The model under review builds one solid part; all positions refer to its coordinate system, in mm. A direction names the side the tool comes from. Give positions to 0.01 mm unless a question says otherwise; leave off trailing zeros. Order: outer loops, then holes, each group sorted by start corner. A loop starts at its lowest first (then second) coordinate and runs counter-clockwise, first axis right, second up. Notation, with made-up numbers: (-32.75, 12.5) - (23.25, 12.5) arc R18 cw to (23.25, 32.5) - close; hole circle Ø4 at (-8.5, 79.5). An arc over 180 degrees is marked (long way). Use CSV: the item, a comma, the result in double quotes.
```python
from build123d import *

# Parameters (mm, degrees)
F0_W     = 12.446
F0_H     = 6.096
F1_DEPTH = 5.715
F2_W     = 12.446
F2_H     = 8.509
F3_DEPTH = 10.414
F4_R     = 0.762
F7_D     = 7.874
F7_DEPTH = 6.605


with BuildPart() as f1:
    # F0 (on Top) → F1 (new body)
    with BuildSketch(Plane.XY):
        Rectangle(F0_W, F0_H)
    extrude(amount=F1_DEPTH)

    # F2 (on Top) → F3 (join)
    with BuildSketch(Plane.XY):
        Rectangle(F2_W, F2_H)
    extrude(amount=-F3_DEPTH)

    # F4
    f4_edges = [f1.edges().sort_by_distance(p)[0] for p in [
        (6.223, 0, 5.715),
        (0, 3.048, 5.715),
        (-6.223, 0, 5.715),
        (0, -3.048, 5.715),
    ]]
    fillet(f4_edges, radius=F4_R)

    # F7 (through all, one way)
    with BuildSketch(Plane.XY.offset(-3.81)):
        with Locations((0, 0)):
            Circle(F7_D / 2)
    extrude(amount=-F7_DEPTH, mode=Mode.SUBTRACT)


solid = f1.part
```
Item 1: Tool access review of faces 5 (the face through (0, -4, 0)), 6 (the face through (0, 4, 0)), 7 (the face through (0, 4.254, -5)): name each direction out of +Z, -Z, +X, -X, +Y, -Y from which nothing blocks a thin tool from reaching the whole face with its end or side.
Results list:
face 5,"+Z, +X, -X, -Y"
face 6,"+Z, +X, -X, +Y"
face 7,"+Z, -Z, +X, -X, +Y"
Item 2: Wall thickness on L1, parallel to Y at x = 0, z = -6.5; L2, parallel to Z at x = -0.5, y = -0.75 (3 decimals); L3, parallel to Z at x = -3, y = -3.25: over which ranges is each line inside the solid? List them lowest first.
Results list:
L1,"y = -4.25 to -3.94, 3.94 to 4.25"
L2,"z = -3.81 to 5.715"
L3,"z = -10.41 to 0"
Item 3: Take a section at A-A, the plane x = 5.25. Give the boundary of the cut face in (y, z) (1 decimal).
Results list:
outline,"(-4.3, -10.4) - (4.3, -10.4) - (4.3, 0) - (3, 0) - (3, 5) arc R0.8 ccw to (2.3, 5.7) - (-2.3, 5.7) arc R0.8 ccw to (-3, 5) - (-3, 0) - (-4.3, 0) - close"
Item 4: Take a section at B-B, the plane y = 0. Give the boundary of the cut face in (x, z) (3 decimals), and give its area (3 significant figures).
Results list:
outline,"(-6.223, -10.414) - (-3.937, -10.414) - (-3.937, -3.81) - (3.937, -3.81) - (3.937, -10.414) - (6.223, -10.414) - (6.223, 4.953) arc R0.762 ccw to (5.461, 5.715) - (-5.461, 5.715) arc R0.762 ccw to (-6.223, 4.953) - close"
area,"148 mm2"
Item 5: Mouldability with a two-part tool opening along Y and no side actions: class faces 1 (the face through (0, 0, -3.81)), 2 (the face through (-0.853, -3.843, -7.066)), 3 (the face through (0, -3.048, 2)), 4 (the face through (0, 0, 5.715)) as pulls with the +Y half, pulls with the -Y half, needs draft (parallel to the pull), parting line crosses it, or undercut.
Results list:
face 1,"undercut"
face 2,"undercut"
face 3,"pulls with the -Y half"
face 4,"needs draft"
Item 6: Clearance check with flat-ended pins moving along their axes: pin 1 (0.6 mm diameter, centred on x = 0, y = 3.5, fed in from +Z); pin 2 (1.5 mm diameter, centred on x = -0.5, z = 2, fed in from +Y); pin 3 (4 mm diameter, centred on x = 0, z = 3.5, fed in from -Y). State where each tip first meets the part, or that it passes through.
Results list:
pin 1,"stops at z = 0"
pin 2,"stops at y = 3.05"
pin 3,"stops at y = -3.05"
Item 7: Take a section at C-C, the plane z = -8.75. Give the boundary of the cut face in (x, y).
Results list:
outline,"(-6.22, -4.25) - (6.22, -4.25) - (6.22, 4.25) - (-6.22, 4.25) - close; hole circle Ø7.87 at (0, 0)"
